For this review, take the finished solid that the model builds, in its own axes (mm). Give positions to 0.01 mm unless a question says otherwise; leave off trailing zeros. Write each loop counter-clockwise with the first axis right and the second up, starting at its lowest first coordinate (ties: lowest second). Pieces come first, ordered by that corner, then holes. Notation, with made-up numbers: M 9,34 L 64,34 A17 cw 64,47 Z; hole C 89.5,78.25 d9. An arc over 180 degrees is marked long. One line per item, written item: value. Start each with the question number.
Item 1: Consider section B-B, the plane z = 0. Write out the cut boundary in (x, y), and give its area (3 significant figures).
Item 2: Consider section C-C, the plane y = -42. Write out the cut boundary in (x, z).
Item 3: To check wall thickness, follow probe 1 along Y at (x, z) = (3.55, 0); probe 2 along Y at (x, z) = (2.85, -34); probe 3 along Y at (x, z) = (1.6, -8). State the ranges of each line that lie inside material, in increasing order.
Item 4: Consider section A-A, the plane y = 0. Write out the cut boundary in (x, z).
Item 5: Consider section D-D, the plane x = 3.2. Write out the cut boundary in (y, z), and give its area (3 significant figures).
Item 6: Clearance check with flat-ended pins moving along their axes: pin 1 Ø2 at (x, y) = (3, 67.5) entering from -Z; pin 2 Ø1.5 at (x, y) = (3.5, -23.5) entering from +Z. State where each tip first meets the part, or that it passes through.
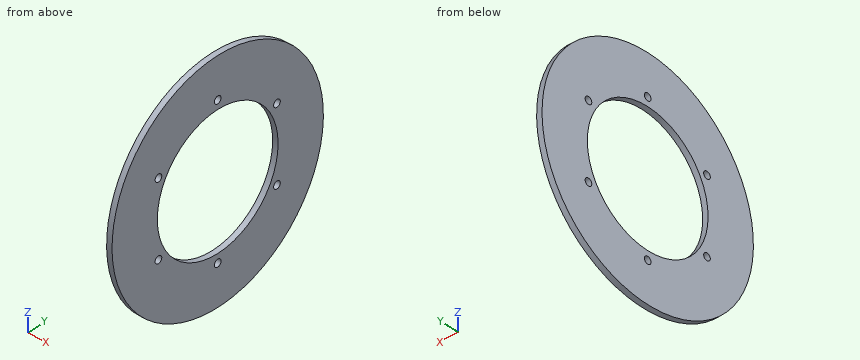
Solid Edge part; units mm, degrees
sketch "Sketch1" plane through (0, 0, 0) normal (0, -1, 0) x (1, 0, 0)
  line L0 (0.073, 60) -> (5.073, 60)
  line L1 (5.073, 60) -> (5.073, 105)
  line L2 (5.073, 105) -> (0.073, 105)
  line L3 (0.073, 105) -> (0.073, 60)
  dimension "D1" = 5.073
  dimension "D2" = 5.073
revolve "RevolvedProtrusion1" add sketch "Sketch1" angle 360 about axis through (23.5691, 0, 0) along (-1, 0, 0)
hole "Hole1" at (5.073, 0, 68) direction (-1, 0, 0) diameter 6.6 end up to next
hole "Hole2" at (5.073, -58.8897, 34) direction (-1, 0, 0) diameter 6.6 end up to next
hole "Hole3" at (5.073, -58.8897, -34) direction (-1, 0, 0) diameter 6.6 end up to next
hole "Hole4" at (5.073, 0, -68) direction (-1, 0, 0) diameter 6.6 end up to next
hole "Hole5" at (5.073, 58.8897, -34) direction (-1, 0, 0) diameter 6.6 end up to next
hole "Hole6" at (5.073, 58.8897, 34) direction (-1, 0, 0) diameter 6.6 end up to next
properties material "Steel"
Model answer:
1. outline: M 0.07,-105 L 5.07,-105 L 5.07,-60 L 0.07,-60 Z; M 0.07,60 L 5.07,60 L 5.07,105 L 0.07,105 Z
1. area: 450 mm2
2. outline: M 0.07,-96.23 L 5.07,-96.23 L 5.07,-42.85 L 0.07,-42.85 Z; M 0.07,42.85 L 5.07,42.85 L 5.07,96.23 L 0.07,96.23 Z
3. probe 1: y = -105 to -60, 60 to 105
3. probe 2: y = -99.34 to -62.19, -55.59 to -49.44, 49.44 to 55.59, 62.19 to 99.34
3. probe 3: y = -104.69 to -59.46, 59.46 to 104.69
4. outline: M 0.07,-105 L 5.07,-105 L 5.07,-71.3 L 0.07,-71.3 Z; M 0.07,-64.7 L 5.07,-64.7 L 5.07,-60 L 0.07,-60 Z; M 0.07,60 L 5.07,60 L 5.07,64.7 L 0.07,64.7 Z; M 0.07,71.3 L 5.07,71.3 L 5.07,105 L 0.07,105 Z
5. outline: C 0,0 d210; hole C -58.89,-34 d6.6; hole C -58.89,34 d6.6; hole C 0,0 d120; hole C 0,-68 d6.6; hole C 0,68 d6.6; hole C 58.89,-34 d6.6; hole C 58.89,34 d6.6
5. area: 23,100 mm2
6. pin 1: stops at z = -81.26
6. pin 2: stops at z = 102.51
